from build123d import *

# Parameters (mm, degrees)
SKETCH1_W           = 76.2
SKETCH1_H           = 135.6868
BOSS_EXTRUDE1_DEPTH = 3.175
SKETCH2_W           = 12.7
SKETCH2_H           = 8.6868
CUT_EXTRUDE1_DEPTH  = 78.874370293
SKETCH3_W           = 12.0904
SKETCH3_H           = 19.05
CUT_EXTRUDE2_DEPTH  = 78.874370293


with BuildPart() as part:
    # Sketch1 → Boss-Extrude1 (new body)
    with BuildSketch(Plane.XY):
        Rectangle(SKETCH1_W, SKETCH1_H)
    extrude(amount=BOSS_EXTRUDE1_DEPTH)

    # Sketch2 → Cut-Extrude1 (cut, through all)
    with BuildSketch(Plane.XY.offset(3.175)):
        with Locations((0, 67.8434)):
            Rectangle(SKETCH2_W, SKETCH2_H)
        with Locations((-25.4, 67.8434)):
            Rectangle(SKETCH2_W, SKETCH2_H)
        with Locations((25.4, 67.8434)):
            Rectangle(SKETCH2_W, SKETCH2_H)
        with Locations((25.4, -67.8434)):
            Rectangle(SKETCH2_W, SKETCH2_H)
        with Locations((-25.4, -67.8434)):
            Rectangle(SKETCH2_W, SKETCH2_H)
        with Locations((0, -67.8434)):
            Rectangle(SKETCH2_W, SKETCH2_H)
    extrude(amount=-CUT_EXTRUDE1_DEPTH, mode=Mode.SUBTRACT)

    # Sketch3 → Cut-Extrude2 (cut, through all)
    with BuildSketch(Plane.XY.offset(3.175)):
        with Locations((38.1, 0)):
            Rectangle(SKETCH3_W, SKETCH3_H)
        with Locations((38.1, 38.1)):
            Rectangle(SKETCH3_W, SKETCH3_H)
        with Locations((38.1, -38.1)):
            Rectangle(SKETCH3_W, SKETCH3_H)
        Polygon((-44.277990322, 28.743505915), (-32.187678137, 28.697425322), (-32.115072161, 47.747286959), (-44.205384346, 47.793367552), align=None)
        Polygon((-32.332890089, -9.402297951), (-32.260284113, 9.647563686), (-44.350596298, 9.693644279), (-44.423202274, -9.356217358), align=None)
        Polygon((-32.405496065, -28.452159587), (-32.478102041, -47.502021224), (-44.568414227, -47.455940631), (-44.495808251, -28.406078995), align=None)
    extrude(amount=-CUT_EXTRUDE2_DEPTH, mode=Mode.SUBTRACT)


solid = part.part
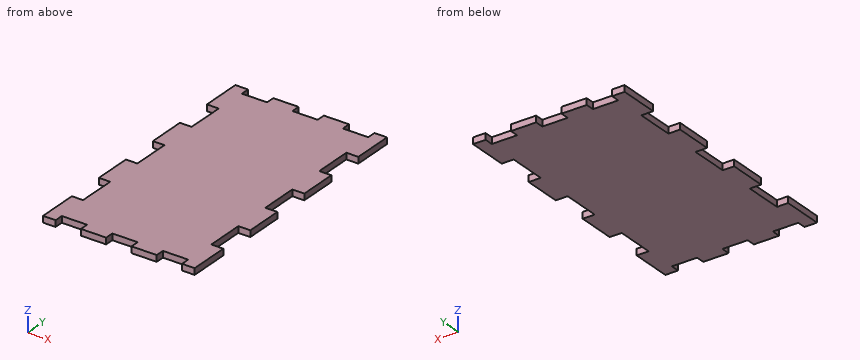
Work out the finished part from the listing and answer in its coordinate system (mm). Coordinates: 2 decimals unless noted, no trailing zeros. Write each loop counter-clockwise with the first axis right and the second up, starting at its lowest first coordinate (ties: lowest second). Pieces come first, ordered by that corner, then holes. Notation, with made-up numbers: M 65,-22 L 77,-22 A35 ccw 77,10 Z; hole C 13.25,8 d4. An arc over 180 degrees is marked long. Answer as CSV lines item,"result". Start each with the question number.
Item 1: Section B-B on y = -6.5 is taken. Write down the section's boundary in (x, z) (3 decimals).
Item 2: Section A-A on x = 24.5 is taken. Write down the section's boundary in (y, z) (3 decimals).
Item 3: Flat-ended cylindrical pins translate along their axes: P1, Ø1.6, axis at x = 1.5, z = 1.5, coming from the +Y side; P2, Ø1, axis at y = -0.5, z = 2, coming from the +X side. Find the tip coordinate at first contact, or state that the pin passes through.
Item 4: Consider L1, parallel to Y at x = -6, z = 0.4; L2, parallel to X at y = 46.5, z = 1.1; L3, parallel to X at y = -1, z = 2.3. Determine where each line is inside the solid, lowest interval first.
Checks:
1,outline,"M -32.322,0 L 32.055,0 L 32.055,3.175 L -32.322,3.175 Z"
2,outline,"M -63.5,0 L 63.5,0 L 63.5,3.175 L -63.5,3.175 Z"
3,P1,"stops at y = 63.5"
3,P2,"stops at x = 32.05"
4,L1,"y = -63.5 to 63.5"
4,L2,"x = -32.12 to 32.05"
4,L3,"x = -32.3 to 32.05"
